Autodesk Inventor part; units mm, degrees
ref_plane "YZ Plane" through (0, 0, 0) normal (1, 0, 0) x (0, 1, 0)
ref_plane "XZ Plane" through (0, 0, 0) normal (0, 1, 0) x (-1, 0, 0)
ref_plane "XY Plane" through (0, 0, 0) normal (0, 0, 1) x (1, 0, 0)
sketch "Sketch1" plane through (0, 0, 0) normal (0, 0, 1) x (1, 0, 0)
  line L0 (0, 0) -> (65, 0) construction
  line L1 (0, -4) -> (65, -4)
  line L2 (65, 4) -> (0, 4)
  arc A0 (0, 4) -> (0, -4) centre (0, 0) ccw
  arc A1 (65, -4) -> (65, 4) centre (65, 0) ccw
  point P0 (32.5, 0)
  dimension "d0" = 65
  dimension "d1" = 4
extrude "Extrusion1" add sketch "Sketch1" against normal blind 3
hole "Hole1" at (0, 0, 0) at (65, 0, 0) direction (0, 0, -1) diameter 3 depth 8 tip angle 118
properties part number "LegBaseLink"
The listing builds one solid part. Answer for the finished solid, in the listing's coordinates (mm). Coordinates: 2 decimals unless noted, no trailing zeros. Loops run counter-clockwise (first coordinate to the right, second up) from the corner with the lowest first, then second, coordinate; pieces in that order, holes last. Notation, with made-up numbers: (70, -32) - (102, -32) arc R26 cw to (102, -7) - close; hole circle Ø10 at (25, 48.5). An arc over 180 degrees is marked (long way). Write item = value, one per line.
1) Determine the mould class of faces 1 (the face through (32, 0, -3)), 2 (the face through (63.513, 0.195, -1.521)), 3 (the face through (-4, 0, -1)), 4 (the face through (-0.07, 1.5, -1.52)) for opening direction X: pulls with the +X half, pulls with the -X half, needs draft (parallel to the pull), parting line crosses it, or undercut.
Responses:
face_1 = needs draft
face_2 = undercut
face_3 = pulls with the -X half
face_4 = undercut
2) Find the intervals of material crossed by line 1 along X through (y, z) = (0, -2.15); line 2 along Y through (x, z) = (65, -0.9); line 3 along X through (y, z) = (-1.25, -2.5), in increasing order.
Responses:
line_1 = -4 to -1.5, 1.5 to 63.5, 66.5 to 69
line_2 = -4 to -1.5, 1.5 to 4
line_3 = -3.8 to -0.83, 0.83 to 64.17, 65.83 to 68.8
3) Section B-B (z = -2.45) is taken. Determine the outline of the cut face in (x, y).
Responses:
outline = (0, -4) - (65, -4) arc R4 ccw to (65, 4) - (0, 4) arc R4 ccw to start; hole circle Ø3 at (0, 0); hole circle Ø3 at (65, 0)
4) Each of these flat-tipped pins is pushed along its axis until it touches: P1, Ø1, axis at y = -1.5, z = -2.5, coming from the -X side; P2, Ø1, axis at y = 2.5, z = -0.5, coming from the +X side; P3, Ø2.5, axis at x = 0, y = 0, coming from the +Z side; P4, Ø1, axis at y = -3, z = -1, coming from the -X side. Where does it stop, or does it pass through?
Responses:
P1 = -3.87
P2 = 68.46
P3 = through
P4 = -3.12
5) Section A-A (y = 0) is taken. Determine the outline of the cut face in (x, z), plus the area to 3 significant figures.
Responses:
outline = (-4, -3) - (-1.5, -3) - (-1.5, 0) - (-4, 0) - close; (1.5, -3) - (63.5, -3) - (63.5, 0) - (1.5, 0) - close; (66.5, -3) - (69, -3) - (69, 0) - (66.5, 0) - close
area = 201 mm^2
